Read the model definition and answer for the solid it produces. Units are mm, in the model's axes. Face numbers are marked on the shaded views. Give positions to 0.01 mm unless a question says otherwise; leave off trailing zeros. Order: outer loops, then holes, each group sorted by start corner. A loop starts at its lowest first (then second) coordinate and runs counter-clockwise, first axis right, second up.
```python
from build123d import *

# Parameters (mm, degrees)
BOSS_EXTRUDE1_DEPTH = 11
BOSS_EXTRUDE2_REACH = 31.074


with BuildPart() as part:
    # Sketch2 → Boss-Extrude1 (new body)
    with BuildSketch(Plane(origin=(0, 0, 0), x_dir=(0, 0, -1), z_dir=(1, 0, 0))):
        Polygon((-7.428495294, -9.782945939), (25.071504706, -9.782945939), (25.071504706, -3.782945939), (-7.428495294, 8.046086675), align=None)
    extrude(amount=-BOSS_EXTRUDE1_DEPTH)

    # Cut-Sweep3: sweep along a path in Sketch5
    with BuildLine(Plane.ZY.offset(11)) as cut_sweep3_path:
        Line((-25.071504706, -6.975479256), (8.757429642, 5.337245904))
    # Sketch3 → Cut-Sweep3 (sweep, cut)
    with BuildSketch(Plane(origin=(0, 0, -25.071504706), x_dir=(-1, 0, 0), z_dir=(0, 0, -1))):
        Polygon((3, -6.782945939), (8, -6.782945939), (7, -3.782945939), (4, -3.782945939), align=None)
    sweep(path=cut_sweep3_path.line, mode=Mode.SUBTRACT)

    # Boss-Extrude2: up to this face of the body (flat: up to its plane)
    boss_extrude2_end = Plane(part.part.faces().sort_by_distance((0, -3.336347692, -6.132602991))[0])
    # Sketch6 → Boss-Extrude2 (add, up to the picked face)
    with BuildSketch(Plane.ZY.offset(11), mode=Mode.PRIVATE) as boss_extrude2_sk1:
        Polygon((5.573598846, 4.37095958), (7.428495294, 5.046086675), (7.428495294, 6.584184475), (4.844649108, 13.683243526), (2.495417556, 12.828193167), align=None)
    boss_extrude2_tool1 = split(extrude(boss_extrude2_sk1.sketch, amount=-BOSS_EXTRUDE2_REACH, mode=Mode.PRIVATE), bisect_by=boss_extrude2_end, keep=Keep.BOTH, mode=Mode.PRIVATE)
    add(boss_extrude2_tool1.solids().sort_by(Axis((-11, 9.08568, 5.168148), (1, 0, 0)))[0])


solid = part.part
```
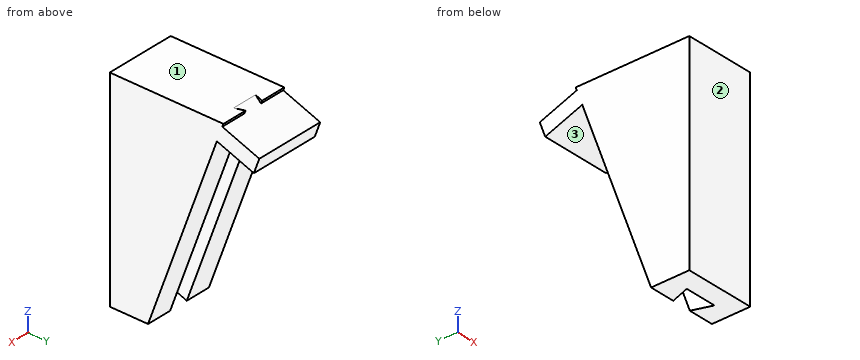
1) The part is cut by section A-A on x = -8.5. Determine the outline of the cut face in (y, z).
Final values:
outline: (-9.78, -25.07) - (-3.78, -25.07) - (7.02, 4.61) - (12.83, 2.5) - (13.68, 4.84) - (7.88, 6.96) - (8.05, 7.43) - (-9.78, 7.43) - close
2) The part is cut by section C-C on x = -6. Determine the outline of the cut face in (y, z), and give its area (3 significant figures).
Final values:
outline: (-9.78, -25.07) - (-6.78, -25.07) - (4.37, 5.57) - (12.83, 2.5) - (13.68, 4.84) - (6.58, 7.43) - (-9.78, 7.43) - close
area: 312 mm2
3) For a pull along Y with two mould halves and no side action, classify the marked faces 1, 2 and 3 as released by +Y, released by -Y, zero draft, split by the parting line, or undercut.
Final values:
face 1: zero draft
face 2: released by -Y
face 3: undercut
4) Given pin 1 (6 mm diameter, centred on x = -8.5, z = -18, fed in from +Y), flat-ended and moving along its own axis, determine where the tip first touches the part or whether it passes through.
Final values:
pin 1: stops at y = -0.12
5) Consider L1, parallel to Y at x = -10.25, z = -22.5; L2, parallel to Y at x = -6.75, z = -4.5; L3, parallel to Z at x = -3, y = 10.5. Determine where each line is inside the solid, lowest interval first.
Final values:
L1: y = -9.78 to -2.85
L2: y = -9.78 to 0.7
L3: z = 3.34 to 6
6) The part is cut by section B-B on y = -4.75. Determine the outline of the cut face in (x, z).
Final values:
outline: (-11, -25.07) - (-7.32, -25.07) - (-8, -19.49) - (-3, -19.49) - (-3.68, -25.07) - (0, -25.07) - (0, 7.43) - (-11, 7.43) - close
